Design review of the part shown in the three views and the two pictorial views. Dimensions are in mm from the part's minimum x, y and z. Give positions to 0.01 mm unless a question says otherwise; leave off trailing zeros. Loops run counter-clockwise (first coordinate to the right, second up) from the corner with the lowest first, then second, coordinate; pieces in that order, holes last. Notation, with made-up numbers: (62, 75.5) -> (82, 75.5) arc R27 cw to (82, 111.5) -> close; hole circle Ø6 at (9.5, 86.25). An arc over 180 degrees is marked (long way). Answer as CSV lines item,"result".
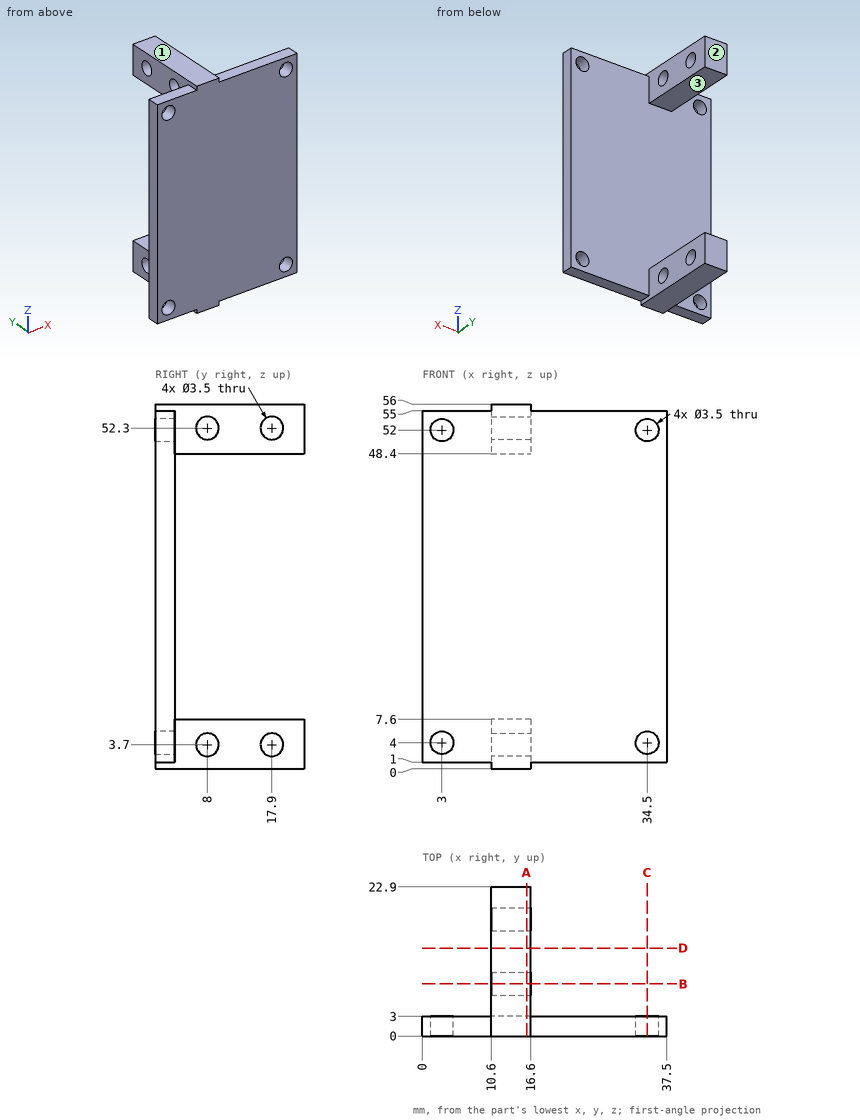
Q1. We need section C-C, the plane x = 34.5. State the section outline as (y, z) points.
Filled sheet:
outline,"(0, 1) -> (3, 1) -> (3, 2.25) -> (0, 2.25) -> close; (0, 5.75) -> (3, 5.75) -> (3, 50.25) -> (0, 50.25) -> close; (0, 53.75) -> (3, 53.75) -> (3, 55) -> (0, 55) -> close"
Q2. We need section B-B, the plane y = 8. State the section outline as (x, z) points, and give its area (3 significant figures).
Filled sheet:
outline,"(10.6, 0) -> (16.6, 0) -> (16.6, 1.95) -> (10.6, 1.95) -> close; (10.6, 5.45) -> (16.6, 5.45) -> (16.6, 7.6) -> (10.6, 7.6) -> close; (10.6, 48.4) -> (16.6, 48.4) -> (16.6, 50.55) -> (10.6, 50.55) -> close; (10.6, 54.05) -> (16.6, 54.05) -> (16.6, 56) -> (10.6, 56) -> close"
area,"49.2 mm^2"
Q3. We need section D-D, the plane y = 13.5. State the section outline as (x, z) points, and give its area (3 significant figures).
Filled sheet:
outline,"(10.6, 0) -> (16.6, 0) -> (16.6, 7.6) -> (10.6, 7.6) -> close; (10.6, 48.4) -> (16.6, 48.4) -> (16.6, 56) -> (10.6, 56) -> close"
area,"91.2 mm^2"
Q4. We need section A-A, the plane x = 16. State the section outline as (y, z) points.
Filled sheet:
outline,"(0, 0) -> (22.9, 0) -> (22.9, 7.6) -> (3, 7.6) -> (3, 48.4) -> (22.9, 48.4) -> (22.9, 56) -> (0, 56) -> close; hole circle Ø3.5 at (8, 3.7); hole circle Ø3.5 at (8, 52.3); hole circle Ø3.5 at (17.9, 3.7); hole circle Ø3.5 at (17.9, 52.3)"
Q5. Clearance check with flat-ended pins moving along their axes: pin 1 Ø4 at (y, z) = (8, 52.3) entering from -X; pin 2 Ø5 at (x, z) = (13, 21) entering from +Y; pin 3 Ø2.5 at (y, z) = (17, 5.5) entering from +X. State where each tip first meets the part, or that it passes through.
Filled sheet:
pin 1,"stops at x = 10.6"
pin 2,"stops at y = 3"
pin 3,"stops at x = 16.6"
Q6. The part is to be moulded in two halves that separate along Z. For the marked faces 1, 2 and 3, say which applies: pulls with the +Z half, pulls with the -Z half, needs draft (parallel to the pull), parting line crosses it, or undercut.
Filled sheet:
face 1,"pulls with the +Z half"
face 2,"needs draft"
face 3,"undercut"
Q7. To check wall thickness, follow probe 1 along Y at (x, z) = (13, 52.3); probe 2 along X at (y, z) = (1.55, 4); probe 3 along Z at (x, y) = (14, 7.5). State the ranges of each line that lie inside material, in increasing order. Write a range as from..to.
Filled sheet:
probe 1,"y = 0..6.25, 9.75..16.15, 19.65..22.9"
probe 2,"x = 0..1.25, 4.75..32.75, 36.25..37.5"
probe 3,"z = 0..2.02, 5.38..7.6, 48.4..50.62, 53.98..56"
